Input: dimensioned drawing with shaded views. Units: mm. Origin: part minimum x, y, z. Round coordinates to 2 decimals unless told otherwise and drop trailing zeros. Loops run counter-clockwise (first coordinate to the right, second up) from the corner with the lowest first, then second, coordinate; pieces in that order, holes last. Notation, with made-up numbers: M 69,59.25 L 76,59.25 A29 ccw 76,82.25 Z; hole C 62,58.25 d4. An arc over 180 degrees is marked long. Return JSON: item names as keys, results as strings.
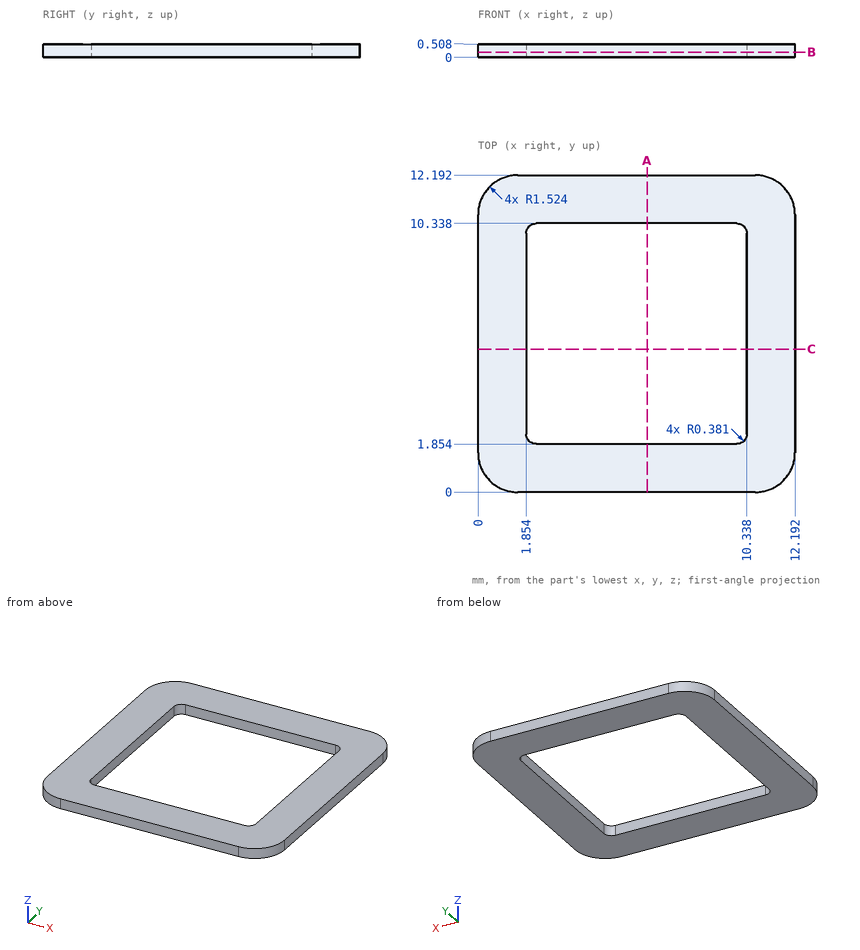
Q1. Section query A-A (x = 6.5). Output: boundary loops of the cut face in (y, z).
Determined:
{"outline": "M 0,0 L 1.85,0 L 1.85,0.51 L 0,0.51 Z; M 10.34,0 L 12.19,0 L 12.19,0.51 L 10.34,0.51 Z"}
Q2. Material intervals for L1, parallel to Y at x = 9, z = 0.4; L2, parallel to X at y = 10.25, z = 0.25, sorted ascending.
Determined:
{"L1": "y = 0 to 1.85, 10.34 to 12.19", "L2": "x = 0 to 1.99, 10.2 to 12.19"}
Q3. Section query B-B (z = 0.2). Output: boundary loops of the cut face in (x, y) (1 decimal), plus the area to 3 significant figures.
Determined:
{"outline": "M 0,1.5 A1.5 ccw 1.5,0 L 10.7,0 A1.5 ccw 12.2,1.5 L 12.2,10.7 A1.5 ccw 10.7,12.2 L 1.5,12.2 A1.5 ccw 0,10.7 Z; hole M 1.9,2.2 A0.4 ccw 2.2,1.9 L 10,1.9 A0.4 ccw 10.3,2.2 L 10.3,10 A0.4 ccw 10,10.3 L 2.2,10.3 A0.4 ccw 1.9,10 Z", "area": "74.8 mm^2"}
